Geometry: final body of the model. Coordinates: model frame, mm. Give positions to 0.01 mm unless a question says otherwise; leave off trailing zeros. Loops run counter-clockwise (first coordinate to the right, second up) from the corner with the lowest first, then second, coordinate; pieces in that order, holes last.
1. Section C-C, the plane x = 78. Output: boundary loops of the cut face in (y, z), then the cut area to 3 significant figures.
2. First-contact query: P1, Ø1.8, axis at x = 1, y = 25, coming from the -Z side; P2, Ø1, axis at x = 25, z = -0.5, coming from the -Y side; P3, Ø1, axis at y = -7.5, z = -3.5, coming from the +X side. Flat tips, straight axial feed; report the tip coordinate or a pass-through.
3. Section B-B, the plane z = -0.7. Output: boundary loops of the cut face in (x, y), then the cut area to 3 significant figures.
4. Section A-A, the plane x = 0.8. Output: boundary loops of the cut face in (y, z), then the cut area to 3 significant figures.
5. Material intervals for line 1 along X through (y, z) = (8, -1.55); line 2 along X through (y, z) = (-15, -3.7); line 3 along Y through (x, z) = (0.8, -2.7), sorted ascending.
from build123d import *

# Parameters (mm, degrees)
RESSALTO_EXTRUS_O1_DEPTH = 48
ESBO_O12_R               = 1.5
CORTE_EXTRUS_O10_DEPTH   = 10
ESBO_O13_R               = 1.5
CORTE_EXTRUS_O11_DEPTH   = 10
ESBO_O14_R               = 1.5
CORTE_EXTRUS_O12_DEPTH   = 10
ESBO_O15_R               = 1.5
CORTE_EXTRUS_O13_DEPTH   = 10
CORTE_EXTRUS_O14_DEPTH   = 10
ESBO_O17_R               = 4
ESBO_O17_W               = 2.8
ESBO_O17_H               = 2.8
RESSALTO_EXTRUS_O2_DEPTH = 4
ESBO_O18_R               = 1.5
RESSALTO_EXTRUS_O3_DEPTH = 4
CHANFRO1_SIZE            = 2
CORTE_EXTRUS_O15_DEPTH   = 48
ESBO_O20_R               = 3
CORTE_EXTRUS_O16_DEPTH   = 2


with BuildPart() as part:
    # Model → Ressalto-extrusão1 (new body)
    with BuildSketch(Plane.XY):
        with BuildLine():
            Line((-0.7, 0), (39, 0))
            Line((39, 0), (39.7, 0))
            Line((39.7, 0), (39.7, -11.380317396))
            Line((39.7, -11.380317396), (50.182424304, -21.8627417))
            Line((50.182424304, -21.8627417), (58.119682605, -29.8))
            Line((58.119682605, -29.8), (81.7, -29.8))
            ThreePointArc((81.7, -29.8), (105.905643752, -13.626305928), (100.226197667, 14.926197667))
            Line((100.226197667, 14.926197667), (65.00338056, 50.149014774))
            Line((65.00338056, 50.149014774), (50.111140335, 50.149014774))
            Line((50.111140335, 50.149014774), (14.181595121, 50.149014774))
            Line((14.181595121, 50.149014774), (-3.2, 32.767419653))
            Line((-3.2, 32.767419653), (-3.2, 5))
            Line((-3.2, 5), (-3.2, 0))
            Line((-3.2, 0), (-0.7, 0))
        make_face()
        with BuildLine():
            Line((-0.7, 2.5), (39, 2.5))
            Line((39, 2.5), (39.7, 2.5))
            Line((39.7, 2.5), (42.2, 2.5))
            Line((42.2, 2.5), (42.2, -10.34478349))
            Line((42.2, -10.34478349), (51.950191257, -20.094974747))
            Line((51.950191257, -20.094974747), (59.15521651, -27.3))
            Line((59.15521651, -27.3), (81.7, -27.3))
            ThreePointArc((81.7, -27.3), (103.595944921, -12.669597347), (98.458430714, 13.158430714))
            Line((98.458430714, 13.158430714), (63.967846654, 47.649014774))
            Line((63.967846654, 47.649014774), (50.111140335, 47.649014774))
            Line((50.111140335, 47.649014774), (15.217129027, 47.649014774))
            Line((15.217129027, 47.649014774), (-0.7, 31.731885747))
            Line((-0.7, 31.731885747), (-0.7, 2.5))
        make_face(mode=Mode.SUBTRACT)
    extrude(amount=RESSALTO_EXTRUS_O1_DEPTH)

    # Esboço12 → Corte-extrusão10 (cut)
    with BuildSketch(Plane(origin=(57.576197667, 57.576197667, 0), x_dir=(0, 0, -1), z_dir=(0.707106781, 0.707106781, 0))):
        with Locations((-44, -19.409915607)):
            Circle(ESBO_O12_R)
        with Locations((-44, -51.409915607)):
            Circle(ESBO_O12_R)
    extrude(amount=-CORTE_EXTRUS_O10_DEPTH, mode=Mode.SUBTRACT)

    # Esboço13 → Corte-extrusão11 (cut)
    with BuildSketch(Plane(origin=(0, 50.149014774, 0), x_dir=(1, 0, 0), z_dir=(0, 1, 0))):
        with Locations((39.59248784, -44)):
            Circle(ESBO_O13_R)
    extrude(amount=-CORTE_EXTRUS_O11_DEPTH, mode=Mode.SUBTRACT)

    # Esboço14 → Corte-extrusão12 (cut)
    with BuildSketch(Plane.ZY.offset(3.2)):
        with Locations((44, 24.383709827)):
            Circle(ESBO_O14_R)
        with Locations((44, 8.383709827)):
            Circle(ESBO_O14_R)
    extrude(amount=-CORTE_EXTRUS_O12_DEPTH, mode=Mode.SUBTRACT)

    # Esboço15 → Corte-extrusão13 (cut)
    with BuildSketch(Plane(origin=(14.159841302, 14.159841302, 0), x_dir=(0, 0, 1), z_dir=(-0.707106781, -0.707106781, 0))):
        with Locations((44, -48.648946546)):
            Circle(ESBO_O15_R)
    extrude(amount=-CORTE_EXTRUS_O13_DEPTH, mode=Mode.SUBTRACT)

    # Esboço16 → Corte-extrusão14 (cut)
    with BuildSketch(Plane.XY.offset(48)):
        Polygon((39.7, 0), (39.7, -2), (42.2, -2), (42.2, 2.5), (-0.7, 2.5), (-0.7, 0), align=None)
    extrude(amount=-CORTE_EXTRUS_O14_DEPTH, mode=Mode.SUBTRACT)

    # Esboço17 → Ressalto-extrusão2 (add)
    with BuildSketch(Plane(origin=(0, 0, 0), x_dir=(-1, 0, 0), z_dir=(0, 0, -1))):
        with Locations((-91.100070488, 18.395470597)):
            Circle(ESBO_O17_R)
        with Locations((-91.100070488, 18.395470597)):
            Rectangle(ESBO_O17_W, ESBO_O17_H, mode=Mode.SUBTRACT)
        with Locations((-68.47265349, 41.022887595)):
            Circle(ESBO_O17_R)
        with Locations((-68.47265349, 41.022887595)):
            Rectangle(ESBO_O17_W, ESBO_O17_H, mode=Mode.SUBTRACT)
        with Locations((-39.59248784, 46.149014774)):
            Circle(ESBO_O17_R)
        with Locations((-39.59248784, 46.149014774)):
            Rectangle(ESBO_O17_W, ESBO_O17_H, mode=Mode.SUBTRACT)
        with Locations((-0.8, 24.383709827)):
            Circle(ESBO_O17_R)
        with Locations((-0.8, 24.383709827)):
            Rectangle(ESBO_O17_W, ESBO_O17_H, mode=Mode.SUBTRACT)
        with Locations((-0.8, 8.383709827)):
            Circle(ESBO_O17_R)
        with Locations((-0.8, 8.383709827)):
            Rectangle(ESBO_O17_W, ESBO_O17_H, mode=Mode.SUBTRACT)
        with Locations((-51.388268427, -17.411731573)):
            Circle(ESBO_O17_R)
        with Locations((-51.388268427, -17.411731573)):
            Rectangle(ESBO_O17_W, ESBO_O17_H, mode=Mode.SUBTRACT)
    extrude(amount=-RESSALTO_EXTRUS_O2_DEPTH)

    # Esboço18 → Ressalto-extrusão3 (add)
    with BuildSketch(Plane(origin=(0, 0, 0), x_dir=(-1, 0, 0), z_dir=(0, 0, -1))):
        with BuildLine():
            Line((-65.00338056, 50.149014774), (-14.181595121, 50.149014774))
            Line((-14.181595121, 50.149014774), (3.2, 32.767419653))
            Line((3.2, 32.767419653), (3.2, 0))
            Line((3.2, 0), (-39.7, 0))
            Line((-39.7, 0), (-39.7, -11.380317396))
            Line((-39.7, -11.380317396), (-58.119682605, -29.8))
            Line((-58.119682605, -29.8), (-81.7, -29.8))
            ThreePointArc((-81.7, -29.8), (-105.905643752, -13.626305928), (-100.226197667, 14.926197667))
            Line((-100.226197667, 14.926197667), (-65.00338056, 50.149014774))
        make_face()
        with Locations((-91.568699638, 17.926841447)):
            Circle(ESBO_O18_R, mode=Mode.SUBTRACT)
        with Locations((-68.47265349, 41.022887595)):
            Circle(ESBO_O18_R, mode=Mode.SUBTRACT)
        with Locations((-39.59248784, 46.149014774)):
            Circle(ESBO_O18_R, mode=Mode.SUBTRACT)
        with Locations((-0.8, 24.383709827)):
            Circle(ESBO_O18_R, mode=Mode.SUBTRACT)
        with Locations((-51.388268427, -17.411731573)):
            Circle(ESBO_O18_R, mode=Mode.SUBTRACT)
        with Locations((-0.8, 8.383709827)):
            Circle(ESBO_O18_R, mode=Mode.SUBTRACT)
    extrude(amount=RESSALTO_EXTRUS_O3_DEPTH)

    # Chanfro1
    chanfro1_edges = [part.edges().sort_by_distance(p)[0] for p in [
        (82.614789114, 32.53760622, -4),
        (105.905643752, -13.626305928, -4),
        (69.909841302, -29.8, -4),
        (48.909841302, -20.590158698, -4),
        (39.7, -5.690158698, -4),
        (18.25, 0, -4),
        (-3.2, 16.383709827, -4),
        (5.49079756, 41.458217213, -4),
        (39.59248784, 50.149014774, -4),
    ]]
    chamfer(chanfro1_edges, length=CHANFRO1_SIZE)

    # Esboço19 → Corte-extrusão15 (cut)
    with BuildSketch(Plane.XY.offset(48)):
        with BuildLine():
            Line((65.00338056, 50.149014774), (14.181595121, 50.149014774))
            Line((14.181595121, 50.149014774), (-3.2, 32.767419653))
            Line((-3.2, 32.767419653), (-3.2, 0))
            Line((-3.2, 0), (39.7, 0))
            Line((39.7, 0), (39.7, -11.380317396))
            Line((39.7, -11.380317396), (58.119682605, -29.8))
            Line((58.119682605, -29.8), (81.7, -29.8))
            ThreePointArc((81.7, -29.8), (105.905643752, -13.626305928), (100.226197667, 14.926197667))
            Line((100.226197667, 14.926197667), (65.00338056, 50.149014774))
        make_face()
    extrude(amount=-CORTE_EXTRUS_O15_DEPTH, mode=Mode.SUBTRACT)

    # Esboço20 → Corte-extrusão16 (cut)
    with BuildSketch(Plane(origin=(0, 0, -4), x_dir=(-1, 0, 0), z_dir=(0, 0, -1))):
        with Locations((-0.8, 24.383709827)):
            Circle(ESBO_O20_R)
        with Locations((-0.8, 8.383709827)):
            Circle(ESBO_O20_R)
        with Locations((-39.59248784, 46.149014774)):
            Circle(ESBO_O20_R)
        with Locations((-68.47265349, 41.022887595)):
            Circle(ESBO_O20_R)
        with Locations((-51.388268427, -17.411731573)):
            Circle(ESBO_O20_R)
        with Locations((-91.568699638, 17.926841447)):
            Circle(ESBO_O20_R)
    extrude(amount=-CORTE_EXTRUS_O16_DEPTH, mode=Mode.SUBTRACT)


solid = part.part
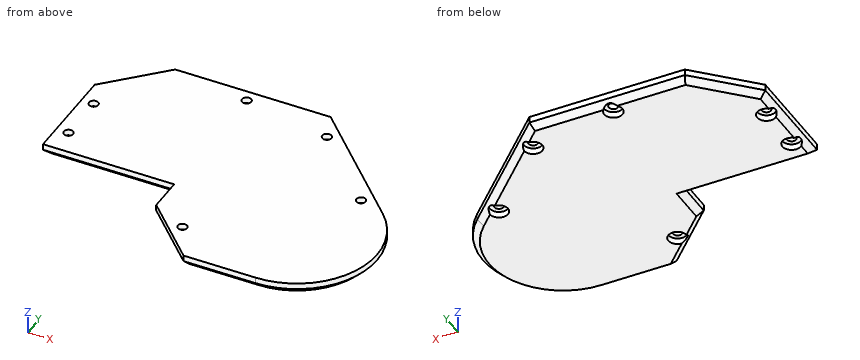
Answers below:
1. outline: (-29.8, -2) - (-27.8, -4) - (34.32, -4) - (37.15, -2) - (37.15, 0) - (-29.8, 0) - close
1. area: 263 mm2
2. P1: stops at z = -2
2. P2: stops at y = 0
2. P3: stops at x = 106.6
3. outline: (-3.2, 0) - (39.7, 0) - (39.7, -11.38) - (58.12, -29.8) - (81.7, -29.8) arc R26.2 ccw to (100.23, 14.93) - (65, 50.15) - (14.18, 50.15) - (-3.2, 32.77) - close; hole circle Ø3 at (0.8, 8.38); hole circle Ø3 at (0.8, 24.38); hole circle Ø3 at (39.59, 46.15); hole circle Ø3 at (51.39, -17.41); hole circle Ø3 at (68.47, 41.02); hole circle Ø3 at (91.57, 17.93)
3. area: 6,160 mm2
4. outline: (0, -2) - (2, -4) - (5.38, -4) - (5.38, -2) - (6.88, -2) - (6.88, 0) - (0, 0) - close; (9.88, -2) - (11.38, -2) - (11.38, -4) - (21.38, -4) - (21.38, -2) - (22.88, -2) - (22.88, 0) - (9.88, 0) - close; (25.88, -2) - (27.38, -2) - (27.38, -4) - (33.94, -4) - (36.77, -2) - (36.77, 0) - (25.88, 0) - close
4. area: 106 mm2
5. line 1: x = -3.2 to -0.65, 2.25 to 105.19
5. line 2: x = 45.72 to 49.6, 53.17 to 103.39
5. line 3: y = 0.7 to 5.38, 11.38 to 21.38, 27.38 to 35.78
